```python
from build123d import *

# Parameters (mm, degrees)
F0_W     = 35
F0_H     = 50
F1_DEPTH = 3.2
F0_H_2   = 1.5
F2_DEPTH = 1.7
F3_DEPTH = 43
F4_R     = 1


with BuildPart() as f1:
    # F0 (on Top) → F1 (new body)
    with BuildSketch(Plane.XY):
        with Locations((19, 79.5)):
            Rectangle(F0_W, F0_H)
        with Locations((19, 26.5)):
            Rectangle(F0_W, F0_H)
    extrude(amount=-F1_DEPTH)

    # F0 (on Top) → F2 (join)
    with BuildSketch(Plane.XY):
        with Locations((19, 53.75)):
            Rectangle(F0_W, F0_H_2)
        Polygon((0, 53), (0, 0), (38, 0), (38, 53), (36.5, 53), (36.5, 51.5), (36.5, 1.5), (1.5, 1.5), (1.5, 51.5), (1.5, 53), align=None)
        with Locations((19, 26.5)):
            Rectangle(F0_W, F0_H)
        with Locations((19, 79.5)):
            Rectangle(F0_W, F0_H)
        with Locations((19, 52.25)):
            Rectangle(F0_W, F0_H_2)
    extrude(amount=F2_DEPTH)

    # F0 (on Top) → F3 (join)
    with BuildSketch(Plane.XY):
        Polygon((0, 106), (0, 53), (1.5, 53), (1.5, 54.5), (1.5, 104.5), (36.5, 104.5), (36.5, 54.5), (36.5, 53), (38, 53), (38, 106), align=None)
        Polygon((0, 53), (0, 0), (38, 0), (38, 53), (36.5, 53), (36.5, 51.5), (36.5, 1.5), (1.5, 1.5), (1.5, 51.5), (1.5, 53), align=None)
    extrude(amount=F3_DEPTH)

    # F4
    f4_edges = [f1.edges().sort_by_distance(p)[0] for p in [
        (0, 0, 21.5),
        (38, 0, 21.5),
        (38, 106, 21.5),
        (0, 106, 21.5),
        (1.5, 104.5, -1.6),
        (36.5, 104.5, -1.6),
        (36.5, 54.5, -1.6),
        (1.5, 54.5, -1.6),
        (1.5, 51.5, -1.6),
        (36.5, 51.5, -1.6),
        (36.5, 1.5, -1.6),
        (1.5, 1.5, -1.6),
    ]]
    fillet(f4_edges, radius=F4_R)


solid = f1.part
```
Geometry check sheet. Reference: the model listing, model coordinates, mm. A direction names the side the tool comes from. Give positions to 0.01 mm unless a question says otherwise; leave off trailing zeros. Write each loop counter-clockwise with the first axis right and the second up, starting at its lowest first coordinate (ties: lowest second). Pieces come first, ordered by that corner, then holes.
1) Gauge pin test, flat ends, axial feed: pin 1 (3.5 mm diameter, centred on y = 86.5, z = -2, fed in from +X); pin 2 (3 mm diameter, centred on x = 12.5, y = 46, fed in from +Z); pin 3 (2.5 mm diameter, centred on x = 14.5, z = -2, fed in from +Y). Record the tip position at first contact, or that the pin passes through.
2) Section check B-B, the plane z = 19. Record the boundary of the cut face in (x, y), and give its area (3 significant figures).
3) Release check for a two-part mould opening along Y. For faces 6 (the flat face through (19, 106, 21)), 7 (the flat face through (36.5, 54, 22)), 8 (the flat face through (1.5, 80, -2)) record: pulls with the +Y half, pulls with the -Y half, needs draft (parallel to the pull), parting line crosses it, or undercut.
4) Access from +Z, -Z, +X, -X, +Y, -Y to the whole of each face (thin tool, end or side, straight path). Record for faces 1 (the flat face through (19, 53, 0)), 2 (the flat face through (19, 1.5, -2)), 3 (the flat face through (1.5, 26, -2)), 4 (the flat face through (19, 1.5, 22)), 5 (the flat face through (19, 104.5, -2)).
5) Material ranges on L1, parallel to X at y = 83, z = 29; L2, parallel to Y at x = 31, z = 25; L3, parallel to Z at x = 27, y = 60, recorded low to high.
6) Section check C-C, the plane y = 18. Record the boundary of the cut face in (x, z), and give its area (4 significant figures).
7) Section check A-A, the plane x = 6. Record the boundary of the cut face in (y, z), and give its area (3 significant figures).
Computed:
1. pin 1: stops at x = 36.5
1. pin 2: stops at z = 1.7
1. pin 3: stops at y = 104.5
2. outline: (0, 1) arc R1 ccw to (1, 0) - (37, 0) arc R1 ccw to (38, 1) - (38, 105) arc R1 ccw to (37, 106) - (1, 106) arc R1 ccw to (0, 105) - close; hole (1.5, 1.5) - (36.5, 1.5) - (36.5, 104.5) - (1.5, 104.5) - close
2. area: 422 mm2
3. face 6: pulls with the +Y half
3. face 7: undercut
3. face 8: needs draft
4. face 1: -Z
4. face 2: -Z, +X, -X, -Y
4. face 3: -Z, -X, +Y, -Y
4. face 4: +Z
4. face 5: -Z, +X, -X, +Y
5. L1: x = 0 to 1.5, 36.5 to 38
5. L2: y = 0 to 1.5, 104.5 to 106
5. L3: z = -3.2 to 1.7
6. outline: (0, 0) - (1.5, 0) - (1.5, -3.2) - (36.5, -3.2) - (36.5, 0) - (38, 0) - (38, 43) - (36.5, 43) - (36.5, 1.7) - (1.5, 1.7) - (1.5, 43) - (0, 43) - close
6. area: 300.5 mm2
7. outline: (0, 0) - (1.5, 0) - (1.5, -3.2) - (51.5, -3.2) - (51.5, 0) - (54.5, 0) - (54.5, -3.2) - (104.5, -3.2) - (104.5, 0) - (106, 0) - (106, 43) - (104.5, 43) - (104.5, 1.7) - (1.5, 1.7) - (1.5, 43) - (0, 43) - close
7. area: 624 mm2
